```python
from build123d import *

# Parameters (mm, degrees)
F5_DEPTH = 25.4
F7_W     = 50.8
F7_H     = 25.4
F8_DEPTH = 50.8


with BuildPart() as f2:
    # F0 (on Front) → F2 (revolve)
    with BuildSketch(Plane.XZ):
        Polygon((56.8157893273, 25.4), (0, 25.4), (-32.0842106727, 25.4), (-57.4842106727, 34.925), (-57.4842106727, 0), (56.8157893273, 0), align=None)
    revolve(axis=Axis((-0.3342106727, 0, 0), (1, 0, 0)))

    # F4 (on Top) → F5 (cut, symmetric)
    with BuildSketch(Plane.XY):
        Polygon((-27.94, -30.9217389812), (58.42, -30.9217389812), (58.42, -17.78), (-3.709944284, -17.78), (-27.94, -25.4), align=None)
    extrude(amount=F5_DEPTH, both=True, mode=Mode.SUBTRACT)

    # F7 (on offset) → F8 (cut)
    with BuildSketch(Plane.XZ.offset(43.18)):
        with Locations((21.690055716, 1.6290084645)):
            Rectangle(F7_W, F7_H)
    extrude(amount=-F8_DEPTH, mode=Mode.SUBTRACT)


solid = f2.part
```
Geometry: final body of the model. Coordinates: model frame, mm. A direction names the side the tool comes from. Round coordinates to 2 decimals unless told otherwise and drop trailing zeros. Order: outer loops, then holes, each group sorted by start corner. A loop starts at its lowest first (then second) coordinate and runs counter-clockwise, first axis right, second up. Notation, with made-up numbers: (-18.5, 62) -> (17.5, 62) arc R8 cw to (17.5, 72) -> close; hole circle Ø10 at (-5, 40.5). An arc over 180 degrees is marked (long way). Use CSV: the item, a comma, the result in double quotes. Start each with the question number.
1) Set-up query: faces 5 (the face through (34, -17.78, -12)), 6 (the face through (11.743, 24.796, -5.506)), 7 (the face through (56.816, 4, 0)), 8 (the face through (21, 7.62, 2)). Return all of +Z, -Z, +X, -X, +Y, -Y with unobstructed straight access to the full face (end or side cutting, diameter ignored); none if empty.
2) Section C-C (x = -1.5). Return the cut outline in (y, z).
3) Section A-A (y = 0). Return the cut outline in (x, z) (3 decimals).
4) Draft query along X for faces 1 (the face through (-57.484, 0, 0)), 2 (the face through (-13, -20.7, 0.3)), 3 (the face through (21, -5, 14.329)), 4 (the face through (47.09, -5, 1)). Return one class per face: +X half, -X half, draft (parallel to the pull), parting line (faces both ways), or undercut.
5) First-contact query: pin 1 Ø10 at (x, y) = (0.5, -5.5) entering from -Z; pin 2 Ø2 at (x, y) = (-1, 9.5) entering from -Z; pin 3 Ø10 at (x, y) = (36, 15) entering from +Z. Flat tips, straight axial feed; report the tip coordinate or a pass-through.
6) Section B-B (z = 0). Return the cut outline in (x, y) (3 decimals), and give its area (3 significant figures).
7) Material intervals for line 1 along X through (y, z) = (5, -2); line 2 along Z through (x, y) = (10.5, 4); line 3 along Y through (x, z) = (30, -0.5), sorted ascending. Write a range as from..to.
Returned:
1,face 5,"+Z, -Z, +X, -Y"
1,face 6,"+X"
1,face 7,"+Z, -Z, +X, +Y, -Y"
1,face 8,"-Y"
2,outline,"(-17.78, -18.14) arc R25.4 ccw (long way) to (-17.78, 18.14) -> (-17.78, 14.33) -> (7.62, 14.33) -> (7.62, -11.07) -> (-17.78, -11.07) -> close"
3,outline,"(-57.484, -34.925) -> (-32.084, -25.4) -> (56.816, -25.4) -> (56.816, 25.4) -> (-32.084, 25.4) -> (-57.484, 34.925) -> close; hole (-3.71, -11.071) -> (47.09, -11.071) -> (47.09, 14.329) -> (-3.71, 14.329) -> close"
4,face 1,"-X half"
4,face 2,"+X half"
4,face 3,"undercut"
4,face 4,"undercut"
5,pin 1,"stops at z = -25.4"
5,pin 2,"stops at z = -23.94"
5,pin 3,"stops at z = 23.35"
6,outline,"(-57.484, -34.925) -> (-32.084, -25.4) -> (-27.94, -25.4) -> (-3.71, -17.78) -> (-3.71, 7.62) -> (47.09, 7.62) -> (47.09, -17.78) -> (56.816, -17.78) -> (56.816, 25.4) -> (-32.084, 25.4) -> (-57.484, 34.925) -> close"
6,area,"4,200 mm²"
7,line 1,"x = -57.48..-3.71, 47.09..56.82"
7,line 2,"z = -25.08..-11.07, 14.33..25.08"
7,line 3,"y = 7.62..25.4"
